Geometry check sheet. Reference: the model listing, model coordinates, mm. Coordinates: 2 decimals unless noted, no trailing zeros. Order: outer loops, then holes, each group sorted by start corner. A loop starts at its lowest first (then second) coordinate and runs counter-clockwise, first axis right, second up. Notation, with made-up numbers: (-40, -14.5) -> (19, -14.5) arc R22 ccw to (19, -7.5) -> close; hole circle Ø9 at (27, 36). An arc over 180 degrees is marked (long way). Answer in a Markdown table with one row per item. Add a question column.
```python
from build123d import *

# Parameters (mm, degrees)
F1_DEPTH = 1.016


with BuildPart() as f1:
    # F0 (on Top) → F1 (new body)
    with BuildSketch(Plane.XY):
        with BuildLine():
            Line((-4.139, 19.660113), (-54.422749, 51.924916))
            Line((-54.422749, 51.924916), (-56.150547, -7.795161))
            ThreePointArc((-56.150547, -7.795161), (-41.837863, -36.389492), (-10.094143, -40.23981))
            Line((-10.094143, -40.23981), (17.741758, -58.094875))
            Line((17.741758, -58.094875), (26.792866, -43.98427))
            Line((26.792866, -43.98427), (4.265871, -29.534551))
            ThreePointArc((4.265871, -29.534551), (9.566227, -19.748967), (11.399325, -8.77212))
            ThreePointArc((11.399325, -8.77212), (7.261307, 7.428431), (-4.139, 19.660113))
        make_face()
    extrude(amount=F1_DEPTH)


solid = f1.part
```
(1) Cross-section at A-A (x = 8). Enter the section's corners in (y, z).
(2) Cross-section at C-C (x = -33). Enter the section's corners in (y, z).
(3) Scan lines: line 1 along Y through (x, z) = (12, 0.6); line 2 along X through (y, z) = (-38, 0.1); line 3 along X through (y, z) = (6.5, 0.3). Record each from-to range of solid material in increasing order.
(4) Mould release check, pull along Y, two halves, no side actions. Record for faces 1 (the face through (-28.929, 35.567, 0.501)), 2 (the face through (15.687, -36.861, 0.501)), 3 (the face through (22.204, -51.138, 0.501)): +Y half, -Y half, draft (parallel to the pull), parting line (faces both ways), or undercut.
(5) Cross-section at D-D (y = 10.5). Enter the section's corners in (x, z), plus the area to 3 significant figures.
(6) Cross-section at B-B (z = 0.85). Enter the section's corners in (x, y), plus the area to 3 significant figures.
(7) Go/stop test with a flat-tipped pin: P1, Ø2, axis at x = 15, y = -42, coming from the -Z side. Record where the tip stops, or that it passes through.
Checks:
| question | item | result |
|---|---|---|
| 1 | outline | (-51.85, 0) -> (-31.93, 0) -> (-31.93, 1.02) -> (-51.85, 1.02) -> close; (-23.54, 0) -> (6, 0) -> (6, 1.02) -> (-23.54, 1.02) -> close |
| 2 | outline | (-40.84, 0) -> (38.18, 0) -> (38.18, 1.02) -> (-40.84, 1.02) -> close |
| 3 | line 1 | -54.41 to -34.5 |
| 3 | line 2 | -39.32 to 17.46 |
| 3 | line 3 | -55.74 to 7.75 |
| 4 | face 1 | +Y half |
| 4 | face 2 | undercut |
| 4 | face 3 | -Y half |
| 5 | outline | (-55.62, 0) -> (5.36, 0) -> (5.36, 1.02) -> (-55.62, 1.02) -> close |
| 5 | area | 62.0 mm² |
| 6 | outline | (-56.15, -7.8) arc R33.78 ccw to (-10.09, -40.24) -> (17.74, -58.09) -> (26.79, -43.98) -> (4.27, -29.53) arc R33.78 ccw to (11.4, -8.77) arc R33.78 ccw to (-4.14, 19.66) -> (-54.42, 51.92) -> close |
| 6 | area | 4,890 mm² |
| 7 | P1 | z = 0 |
